from build123d import *

# Parameters (mm, degrees)
SKETCH_1_W             = 30
SKETCH_1_H             = 15
SM_BASE_FLANGE_1_DEPTH = 1.5
SKETCH_6_R             = 2.5
EXTRUDE_1_DEPTH        = 15
SKETCH_7_R             = 1.5
CUT_EXTRUDE_1_DEPTH    = 15
FILLET_1_R             = 1


# Sheet-metal steps are written as plain solids
with BuildPart() as part:
    # Sketch 1 → 基体-法兰1 (new body)
    with BuildSketch(Plane.XY):
        Rectangle(SKETCH_1_W, SKETCH_1_H)
    extrude(amount=-SM_BASE_FLANGE_1_DEPTH)

    # 草图6 → 凸台-拉伸1 (add)
    with BuildSketch(Plane(origin=(15, 0, 0), x_dir=(0, 0, -1), z_dir=(1, 0, 0))):
        with Locations((2.5, 7.5)):
            Circle(SKETCH_6_R)
    extrude(amount=-EXTRUDE_1_DEPTH)

    # 草图7 → 切除-拉伸1 (cut)
    with BuildSketch(Plane.XY):
        Circle(SKETCH_7_R)
    extrude(amount=-CUT_EXTRUDE_1_DEPTH, mode=Mode.SUBTRACT)

    # 圆角1
    fillet_1_edges = [part.edges().sort_by_distance(p)[0] for p in [
        (15, -7.5, -0.75),
        (-15, -7.5, -0.75),
        (-15, 7.5, -0.75),
    ]]
    fillet(fillet_1_edges, radius=FILLET_1_R)


solid = part.part
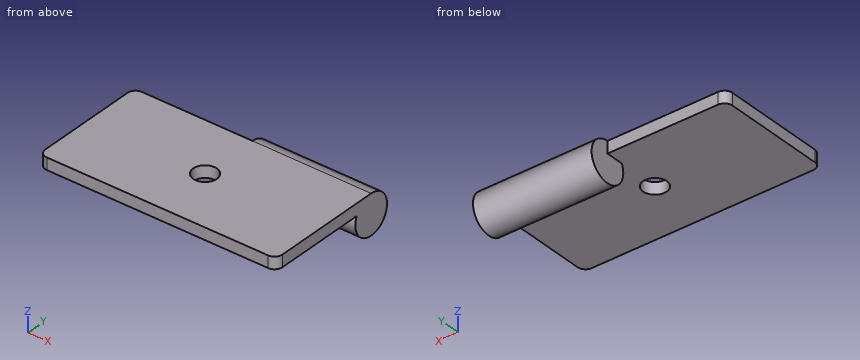
Input: part model. Units: mm. Frame: model coordinates. Give positions to 0.01 mm unless a question says otherwise; leave off trailing zeros. Loops run counter-clockwise (first coordinate to the right, second up) from the corner with the lowest first, then second, coordinate; pieces in that order, holes last. Notation, with made-up numbers: M -24,89.25 L 23,89.25 A23 cw 23,124.25 Z; hole C 48,13 d8. An arc over 180 degrees is marked long. Use one line per item in the form item = value.
1. Section query D-D, the plane z = -2.5. Return the cut outline in (x, y).
Numbers:
outline = M 0,5 L 15,5 L 15,10 L 0,10 Z
2. Section query A-A, the plane y = 0. Return the cut outline in (x, z), and give its area (3 significant figures).
Numbers:
outline = M -15,-1.5 L -1.5,-1.5 L -1.5,0 L -15,0 Z; M 1.5,-1.5 L 15,-1.5 L 15,0 L 1.5,0 Z
area = 40.5 mm²
3. Section query B-B, the plane z = -1.15. Return the cut outline in (x, y), and give its area (3 significant figures).
Numbers:
outline = M -15,-6.5 A1 ccw -14,-7.5 L 14,-7.5 A1 ccw 15,-6.5 L 15,9.6 L 0,9.6 L 0,7.5 L -14,7.5 A1 ccw -15,6.5 Z; hole C 0,0 d3
area = 474 mm²
4. First-contact query: pin 1 (3.5 mm diameter, centred on x = 0, y = 0, fed in from -Z); pin 2 (3 mm diameter, centred on x = 3.5, y = -2.5, fed in from +Z); pin 3 (1.5 mm diameter, centred on x = 9, z = -3.5, fed in from +Y); pin 4 (0.8 mm diameter, centred on x = -7, z = -0.5, fed in from +Y). Flat tips, straight axial feed; report the tip coordinate or a pass-through.
Numbers:
pin_1 = -1.5
pin_2 = 0
pin_3 = 9.99
pin_4 = 7.5
5. Line query: L1, parallel to Z at x = 2.5, y = -6.5; L2, parallel to Y at x = 6.5, z = -2.4; L3, parallel to Y at x = -7, z = -0.25. Output: solid intervals per line, ascending.
Numbers:
L1 = -1.5 to 0
L2 = 5 to 10
L3 = -7.5 to 7.5
6. Section query C-C, the plane y = 2. Return the cut outline in (x, z), and give its area (3 significant figures).
Numbers:
outline = M -15,-1.5 L 15,-1.5 L 15,0 L -15,0 Z
area = 45.0 mm²
